Design review of the part built by this model. Coordinates are the model's own, in mm. A direction names the side the tool comes from. Coordinates: 2 decimals unless noted, no trailing zeros. Loops run counter-clockwise (first coordinate to the right, second up) from the corner with the lowest first, then second, coordinate; pieces in that order, holes last. Notation, with made-up numbers: M 82,27 L 134,27 A15 ccw 134,40 Z; hole C 12,-39.5 d5. An arc over 180 degrees is marked long. Answer as CSV lines item,"result". Start each with the question number.
Autodesk Inventor part; units mm, degrees
ref_plane "YZ Plane" through (0, 0, 0) normal (1, 0, 0) x (0, 1, 0)
ref_plane "XZ Plane" through (0, 0, 0) normal (0, 1, 0) x (-1, 0, 0)
ref_plane "XY Plane" through (0, 0, 0) normal (0, 0, 1) x (1, 0, 0)
sketch "Sketch2" plane through (0, 0, 0) normal (0, 1, 0) x (-1, 0, 0)
  circle A0 centre (0, 0) radius 14
  line L0 (0, 0) -> (0, 14) construction
  line L1 (0, 0) -> (12.1244, -7) construction
  line L2 (0, 0) -> (-12.1244, -7) construction
  circle A1 centre (0, 0) radius 3
  line L3 (2.8191, -1.0261) -> (13.1557, -4.7883)
  line L4 (2.2981, -1.9284) -> (10.7246, -8.999)
  line L5 (0.5209, 2.9544) -> (2.4311, 13.7873)
  line L6 (-0.5209, 2.9544) -> (-2.4311, 13.7873)
  line L7 (-2.8191, -1.0261) -> (-13.1557, -4.7883)
  line L8 (-2.2981, -1.9284) -> (-10.7246, -8.999)
  circle A2 centre (0, 0) radius 16
  circle A3 centre (0, 0) radius 1.8196
  dimension "d10" = 120
  dimension "d11" = 120
  dimension "d18" = 6
  dimension "d19" = 10
  dimension "d20" = 20
  dimension "d21" = 10
  dimension "d22" = 20
  dimension "d23" = 10
  dimension "d24" = 20
  dimension "d26" = 3.6391
  dimension "d29" = 32
  dimension "d30" = 2
extrude "Extrusion1" add sketch "Sketch2" along normal blind 6.6 contours L5 A1 L6 A0 | A0 L4 A1 L3 | A1 | L7 A1 L8 A0 | A2
sketch "Sketch3" plane through (0, 6.6, 0) normal (0, 1, 0) x (1, 0, 0)
  circle A0 centre (0, 0) radius 3
  circle A1 centre (0, 0) radius 1.8196
  circle A2 centre (0, 0) radius 1.8196
extrude "Extrusion2" add sketch "Sketch3" along normal blind 2
fillet "Fillet4" radius 2.54 2 edges at (16, 6.6, 0) (16, 0, 0)
properties part number "wheel"
Item 1: Add section C-C (z = 6.5). Give the number of separate pieces and of enclosed holes in the cut face, plus the area to 3 significant figures.
Item 2: Add section D-D (y = 1.5). Give the boundary of the cut face in (x, z), plus the area to 3 significant figures.
Item 3: For faces 1 (the face through (-1, 0, 2)), 2 (the face through (0, 6.6, 9)), 3 (the face through (12.21, 3.25, 6.85)), list the 3-axis set-ups (+Z, -Z, +X, -X, +Y, -Y) from which the entire face can be reached by the end or side of a thin tool; tool diameter is ignored.
Item 4: For pin 1 (3.5 mm diameter, centred on x = -0.5, z = 7, fed in from +Y); pin 2 (5 mm diameter, centred on x = 1.5, y = 1.5, fed in from +Z); pin 3 (1.5 mm diameter, centred on y = 4.5, z = 5.5, fed in from +X); pin 4 (1 mm diameter, centred on x = 12, y = 2.5, fed in from -Z), all flat-tipped, find the tip position at first contact; note any pin that passes through.
Item 5: Mouldability with a two-part tool opening along Z and no side actions: class faces 4 (the face through (-7.915, 3.254, -2.881)), 5 (the face through (0, 8.6, 2)), 6 (the face through (-0.12, 4.24, -1.816)), 7 (the face through (3.47, 3.29, 15.62)) as released by +Z, released by -Z, zero draft, split by the parting line, or undercut.
Item 6: Add section B-B (y = 5). Give the boundary of the cut face in (x, z), plus the area to 3 significant figures.
Item 7: For line 1 along Z through (x, y) = (0, 3.5); line 2 along Z through (x, y) = (-4, 3.5); line 3 along X through (y, z) = (3, -0.5), list the stretches that pass through material, from the lowest coordinate up. Write a range as from..to.
Item 8: Add section A-A (x = 0). Give the boundary of the cut face in (y, z).
Response:
1,separate pieces,"3"
1,enclosed holes,"0"
1,area,"38.4 mm²"
2,outline,"C 0,0 d31.55; hole M -13.16,-4.79 L -2.82,-1.03 A3 cw -0.52,2.95 L -2.43,13.79 A14 ccw Z; hole M -10.72,-9 A14 ccw 10.72,-9 L 2.3,-1.93 A3 cw -2.3,-1.93 Z; hole C 0,0 d3.64; hole M 0.52,2.95 A3 cw 2.82,-1.03 L 13.16,-4.79 A14 ccw 2.43,13.79 Z"
2,area,"282 mm²"
3,face 1,"+Z, -Z, +X, -X, -Y"
3,face 2,"+Z, +X, -X, +Y"
3,face 3,"+Y, -Y"
4,pin 1,"y = 6.6"
4,pin 2,"z = 16"
4,pin 3,"x = 15.26"
4,pin 4,"z = -11.12"
5,face 4,"undercut"
5,face 5,"zero draft"
5,face 6,"undercut"
5,face 7,"split by the parting line"
6,outline,"C 0,0 d31.64; hole M -13.16,-4.79 L -2.82,-1.03 A3 cw -0.52,2.95 L -2.43,13.79 A14 ccw Z; hole M -10.72,-9 A14 ccw 10.72,-9 L 2.3,-1.93 A3 cw -2.3,-1.93 Z; hole C 0,0 d3.64; hole M 0.52,2.95 A3 cw 2.82,-1.03 L 13.16,-4.79 A14 ccw 2.43,13.79 Z"
6,area,"286 mm²"
7,line 1,"-16..-14, -3..-1.82, 1.82..16"
7,line 2,"-15.49..-13.42, -3.36..-1.46, 13.42..15.49"
7,line 3,"-15.99..-13.99, -2.96..-1.75, 1.75..2.96, 13.99..15.99"
8,outline,"M 0,-3 L 8.6,-3 L 8.6,-1.82 L 0,-1.82 Z; M 0,1.82 L 8.6,1.82 L 8.6,3 L 6.6,3 L 6.6,13.46 A2.54 ccw 4.06,16 L 2.54,16 A2.54 ccw 0,13.46 Z; M 0.06,-14 A2.54 ccw 2.54,-16 L 4.06,-16 A2.54 ccw 6.54,-14 Z"
